Read the model definition and answer for the solid it produces. Units are mm, in the model's axes. A direction names the side the tool comes from. Coordinates: 2 decimals unless noted, no trailing zeros. Write each loop counter-clockwise with the first axis right and the second up, starting at its lowest first coordinate (ties: lowest second). Pieces come first, ordered by that corner, then holes.
from build123d import *

# Parameters (mm, degrees)
VENT_EDGE_BREAK_SIZE = 0.127
FILLET1_R            = 0.254


with BuildPart() as part:
    # Sketch2 → Revolve1 (revolve)
    with BuildSketch(Plane.XY, mode=Mode.PRIVATE) as revolve1_sk:
        Polygon((3.6322, 4.5085), (3.6322, 3.175), (1.27, 3.175), (1.27, 4.5085), (0, 4.5085), (0, 0), (12.9794, 0), (12.9794, 4.5085), (11.7094, 4.5085), (11.7094, 3.175), (9.3472, 3.175), (9.3472, 4.5085), (8.0772, 4.5085), (8.0772, 1.905), (4.9022, 1.905), (4.9022, 4.5085), align=None)
    revolve(revolve1_sk.sketch.rotate(Axis((-1.617419624, 0, 0), (1, 0, 0)), 90), axis=Axis((-1.617419624, 0, 0), (1, 0, 0)))

    # vent-edge-break
    vent_edge_break_edges = [part.edges().sort_by_distance(p)[0] for p in [
        (1.27, 0, -4.5085),
        (3.6322, 0, -4.5085),
        (4.9022, 0, -4.5085),
        (8.0772, 0, -4.5085),
        (9.3472, 0, -4.5085),
        (11.7094, 0, -4.5085),
        (12.9794, 0, -4.5085),
        (0, 0, -4.5085),
    ]]
    chamfer(vent_edge_break_edges, length=VENT_EDGE_BREAK_SIZE)

    # Fillet1
    fillet1_edges = [part.edges().sort_by_distance(p)[0] for p in [
        (4.9022, 0, -1.905),
        (8.0772, 0, -1.905),
    ]]
    fillet(fillet1_edges, radius=FILLET1_R)


solid = part.part
Item 1: The part is cut by section A-A (x = 10). Give the vertices of the cut face in (y, z) (3 decimals), and give its area (3 significant figures).
Item 2: For faces 5 (the flat face through (8.077, 2, 2)), 6 (the cylindrical face through (8.71, 4.4, -0.98)), determine the directions among +Z, -Z, +X, -X, +Y, -Y from which every point of the face is accessible in a straight line to the end or side of a thin tool.
Item 3: Given pin 1 (5 mm diameter, centred on x = 6, z = 3, fed in from -Y); pin 2 (2 mm diameter, centred on x = 10.5, z = -0.5, fed in from +Y) (3 decimals); pin 3 (1 mm diameter, centred on x = 5, z = -2.5, fed in from +Y), each flat-ended and moving along its own axis, determine where each tip first touches the part or whether it passes through.
Item 4: The part is cut by section B-B (x = 4.5). Give the vertices of the cut face in (y, z), and give its area (3 significant figures).
Item 5: Determine the mould class of faces 1 (the flat face through (3.632, -3, 2)), 2 (the flat face through (0, 0, 0)), 3 (the flat face through (4.902, 2, -2)), 4 (the cylindrical face through (12.34, 4.4, -0.98)) for opening direction X: +X half, -X half, draft (parallel to the pull), parting line (faces both ways), or undercut.
Item 6: Find the intervals of material crossed by probe 1 along X at (y, z) = (4, 1.75); probe 2 along X at (y, z) = (-2.5, -1.5); probe 3 along Y at (x, z) = (9.75, 0) (3 decimals), in increasing order.
Answer:
1. outline: circle Ø6.35 at (0, 0)
1. area: 31.7 mm2
2. face 5: none
2. face 6: +X, -X
3. pin 1: stops at y = -4.43
3. pin 2: stops at y = 3.175
3. pin 3: stops at y = 4.01
4. outline: circle Ø9.02 at (0, 0)
4. area: 63.9 mm2
5. face 1: undercut
5. face 2: -X half
5. face 3: undercut
5. face 4: draft
6. probe 1: x = 0 to 1.27, 3.63 to 4.9, 8.08 to 9.35, 11.71 to 12.98
6. probe 2: x = 0 to 4.9, 8.08 to 12.98
6. probe 3: y = -3.175 to 3.175
